Part model, mm, in its own coordinate system. Face numbers are marked on the shaded views. A direction names the side the tool comes from. Round coordinates to 2 decimals unless told otherwise and drop trailing zeros. Loops run counter-clockwise (first coordinate to the right, second up) from the corner with the lowest first, then second, coordinate; pieces in that order, holes last. Notation, with made-up numbers: (78.25, 59.5) -> (127.25, 59.5) arc R27 cw to (127.25, 88.5) -> close; hole circle Ø3 at (1, 74). An arc over 180 degrees is marked (long way). Answer as CSV lines item,"result".
from build123d import *


with BuildPart() as part:
    # Sketch 1 → Revolve 1 (revolve)
    with BuildSketch(Plane.XY, mode=Mode.PRIVATE) as revolve_1_sk:
        with BuildLine():
            Line((288, 0), (288, 7.8))
            ThreePointArc((288, 7.8), (288.087867966, 7.587867966), (288.3, 7.5))
            Line((288.3, 7.5), (298, 7.5))
            Line((298, 7.5), (298, 7.3))
            ThreePointArc((298, 7.3), (298.087867966, 7.087867966), (298.3, 7))
            Line((298.3, 7), (354.533333333, 7))
            Line((354.533333333, 7), (355, 6.533333333))
            Line((355, 6.533333333), (355, 0))
            Line((355, 0), (288, 0))
        make_face()
    revolve(revolve_1_sk.sketch.rotate(Axis((355, 0, 0), (-1, 0, 0)), 270), axis=Axis((355, 0, 0), (-1, 0, 0)))

    # Sketch 2 → Revolve 2 (revolve)
    with BuildSketch(Plane.XY, mode=Mode.PRIVATE) as revolve_2_sk:
        Polygon((0, 0), (0, 10), (120, 10), (121.732050808, 9), (198.267949192, 9), (200, 10), (288, 10), (288, 0), align=None)
    revolve(revolve_2_sk.sketch.rotate(Axis((288, 0, 0), (-1, 0, 0)), 270), axis=Axis((288, 0, 0), (-1, 0, 0)))

    # Sketch 3 → Cut-Revolve 1 (revolve, cut)
    with BuildSketch(Plane.XY, mode=Mode.PRIVATE) as cut_revolve_1_sk:
        Polygon((0, 0), (0, 5), (0.812, 4.188), (24, 4.188), (26.417942927, 0), align=None)
    revolve(cut_revolve_1_sk.sketch.rotate(Axis((26.417942927, 0, 0), (-1, 0, 0)), 270), axis=Axis((26.417942927, 0, 0), (-1, 0, 0)), mode=Mode.SUBTRACT)


solid = part.part
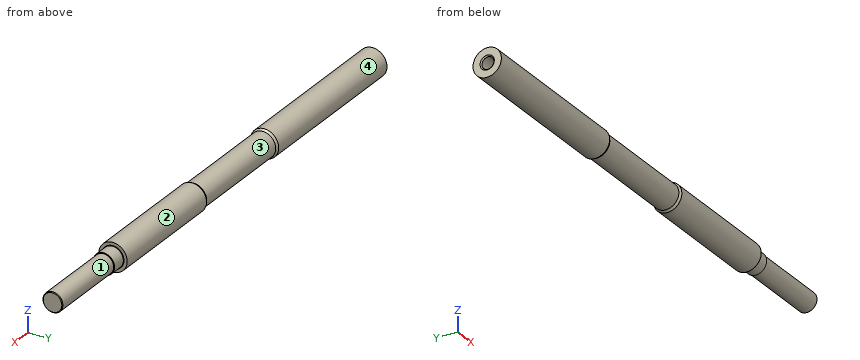
Q1. Saw through at A-A, the plane x = 205. Write the cut outline in (y, z).
Geometry results:
outline,"circle Ø20 at (0, 0)"
Q2. Drill centre lines: line 1 along Y through (x, z) = (18.5, 0); line 2 along Z through (x, y) = (22.5, 0.75); line 3 along X through (y, z) = (3.5, 6.5). Where is each one in solid material? Low to high.
Geometry results:
line 1,"-10 to -4.19, 4.19 to 10"
line 2,"-9.97 to -4.12, 4.12 to 9.97"
line 3,"0 to 298"
Q3. Which spindle directions (+Z, -Z, +X, -X, +Y, -Y) get a long thin tool onto all of the face, cutting with end or side? Do the marked faces 1 and 2. Say none if no direction does.
Geometry results:
face 1,"+X"
face 2,"+X, -X"
Q4. Drop flat-ended pins along their axis: P1, Ø10, axis at x = 112.5, z = -2.5, coming from the +Y side; P2, Ø2, axis at x = 106, y = -5.5, coming from the +Z side; P3, Ø5, axis at y = -0.5, z = -1, coming from the -X side; P4, Ø3, axis at x = 106, y = 2, coming from the -Z side. Give the stop position or say it passes through.
Geometry results:
P1,"y = 10"
P2,"z = 8.93"
P3,"x = 24.33"
P4,"z = -9.99"
Q5. Two-plate mould, pull along X, no slides. Class the marked faces 3 and 4: pulls with the +X half, pulls with the -X half, needs draft (parallel to the pull), parting line crosses it, or undercut.
Geometry results:
face 3,"undercut"
face 4,"needs draft"
